```python
from build123d import *

# Parameters (mm, degrees)
F0_R     = 12.5
F1_DEPTH = 12.5
F2_R     = 12.49999
F3_R     = 11.3
F4_DEPTH = 12.5
F5_SIZE  = 0.5


# Not quite as in the source:
# - a fillet or chamfer is up to 0.001 mm smaller than in the source, because OpenCascade refuses the exact size


with BuildPart() as f1:
    # F0 (on Top) → F1 (new body)
    with BuildSketch(Plane.XY):
        Circle(F0_R)
    extrude(amount=F1_DEPTH)

    # F2 (radius 12.5 in the source; OpenCascade refuses exactly that, so slightly less here)
    f2_edges = [f1.edges().sort_by_distance(p)[0] for p in [
        (-12.5, 0, 12.5),
    ]]
    fillet(f2_edges, radius=F2_R)

    # F3 (on Top) → F4 (join)
    with BuildSketch(Plane.XY):
        Circle(F3_R)
    extrude(amount=-F4_DEPTH)

    # F5
    f5_edges = [f1.edges().sort_by_distance(p)[0] for p in [
        (-11.3, 0, -12.5),
    ]]
    chamfer(f5_edges, length=F5_SIZE)


solid = f1.part
```
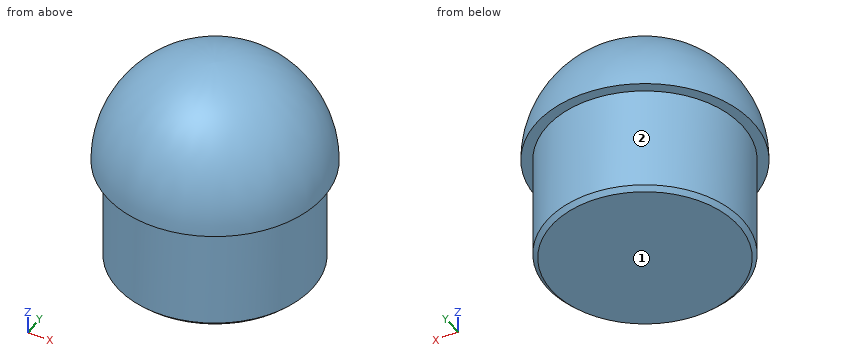
Geometry check sheet. Reference: the model listing, model coordinates, mm. Face numbers are marked on the shaded views. A direction names the side the tool comes from. Give positions to 0.01 mm unless a question says otherwise; leave off trailing zeros.
1) Material ranges on L1, parallel to X at y = 0.25, z = -7; L2, parallel to Y at x = -9, z = -0.75; L3, parallel to X at y = 8, z = -4.25, recorded low to high.
2) Gauge pin test, flat ends, axial feed: pin 1 (1 mm diameter, centred on x = -9.5, y = 3.5, fed in from +Z); pin 2 (5 mm diameter, centred on y = 1, z = -6.5, fed in from -X); pin 3 (6 mm diameter, centred on x = 2.5, z = -2.5, fed in from +Y); pin 4 (12 mm diameter, centred on y = 0.5, z = -5.5, fed in from -X). Record the tip position at first contact, or that the pin passes through.
3) Access from +Z, -Z, +X, -X, +Y, -Y to the whole of each face (thin tool, end or side, straight path). Record for the marked faces 1 and 2.
Computed:
1. L1: x = -11.3 to 11.3
1. L2: y = -6.83 to 6.83
1. L3: x = -7.98 to 7.98
2. pin 1: stops at z = 7.98
2. pin 2: stops at x = -11.3
2. pin 3: stops at y = 12.47
2. pin 4: stops at x = -12.5
3. face 1: -Z, +X, -X, +Y, -Y
3. face 2: -Z
